Read the model definition and answer for the solid it produces. Units are mm, in the model's axes. A direction names the side the tool comes from. Round coordinates to 2 decimals unless told otherwise and drop trailing zeros. Write each loop counter-clockwise with the first axis right and the second up, starting at its lowest first coordinate (ties: lowest second). Pieces come first, ordered by that corner, then holes. Notation, with made-up numbers: (69.5, -13) - (117.5, -13) arc R8 ccw to (117.5, -6) - close; hole circle Ø6 at (59, -1.5). An arc over 180 degrees is marked (long way). Answer as CSV lines item,"result". Start each with the question number.
1) Find section C-C on x = 6. Determine the outline of the cut face in (y, z), then the cut area to 3 significant figures.
2) Each of these flat-tipped pins is pushed along its axis until it touches: pin 1 (2 mm diameter, centred on x = 5.5, y = -3, fed in from -Z); pin 2 (12 mm diameter, centred on y = 3.5, z = -15, fed in from +X). Where does it stop, or does it pass through?
3) Find section D-D on z = -14. Determine the outline of the cut face in (x, y), then the cut area to 3 significant figures.
4) Consider line 1 along X through (y, z) = (-2, 0.4); line 2 along Z through (x, y) = (7.25, -2.75); line 3 along Y through (x, z) = (3.25, -16.75). Determine where each line is inside the solid, lowest interval first.
5) Which of the six approach directions +Z, -Z, +X, -X, +Y, -Y give full straight-line access (tool end or side, diameter ignored) to faces 1 (the cylindrical face through (0.14, 9.43, 0.4)), 2 (the flat face through (0, 9, -10))?
6) For a pull along X with two mould halves and no side action, classify faces 3 (the cylindrical face through (1.952, -1.566, 0.493)), 4 (the flat face through (7.5, -7.5, 0.5)), 5 (the flat face through (0, 1, 0)), 6 (the flat face through (-7.5, -7.5, 0.5)) as +X half, -X half, draft (parallel to the pull), parting line (faces both ways), or undercut.
7) Find section B-B on y = -2. Determine the outline of the cut face in (x, z), then the cut area to 3 significant figures.
8) Find section A-A on x = 0. Determine the outline of the cut face in (y, z).
Autodesk Inventor part; units mm, degrees
ref_plane "YZ Plane" through (0, 0, 0) normal (1, 0, 0) x (0, 1, 0)
ref_plane "XZ Plane" through (0, 0, 0) normal (0, 1, 0) x (-1, 0, 0)
ref_plane "XY Plane" through (0, 0, 0) normal (0, 0, 1) x (1, 0, 0)
sketch "Sketch1" plane through (0, 0, 0) normal (0, 0, 1) x (1, 0, 0)
  line L0 (-10, -10) -> (10, -10)
  line L1 (10, -10) -> (10, 10)
  line L2 (10, 10) -> (-10, 10)
  line L3 (-10, 10) -> (-10, -10)
  line L4 (-10, -10) -> (10, 10) construction
  line L5 (10, -10) -> (-10, 10) construction
  point P0 (0, 0)
  dimension "d0" = 20
  dimension "d1" = 20
extrude "Plate1" add sketch "Sketch1" along normal blind 1
sketch "Sketch2" plane through (10, 9, 1) normal (0, 1, 0) x (-1, 0, 0)
  line L0 (20, 0) -> (0, 0)
  line L1 (0, 0) -> (0, -20)
  line L2 (0, -20) -> (20, -20)
  line L3 (20, -20) -> (20, 0)
edge flange "Flange1" height 20 angle 90 thickness 1 bend radius 1 thickness toward (0, 1, 0) relief tear relief width 1 relief depth 0.5 edges at (0, 10, 0) wall of the first edge with corners at (-10, 9, 1) (10, 9, 1) (10, 9, -19) (-10, 9, -19)
bend "Bend1"
corner "Corner1"
sketch "Sketch3" plane through (0, 0, 1) normal (0, 0, 1) x (1, 0, 0)
  line L0 (5, -10) -> (-5, -10)
  point P0 (0, -2)
  point P1 (0, -2)
  point P2 (10, -10)
  point P3 (-10, -10)
  point P4 (0, -10)
  dimension "d23" = 8
chamfer "Corner Chamfer1" distance 5 angle 45 2 edges at (10, -10, 0.5) (-10, -10, 0.5)
hole "Hole1" at (0, -2, 1) direction (0, 0, -1) diameter 4 depth 1 tip angle 118
equation "\"d21\" = Thickness"
equation "\"d3\" = BendReliefWidth"
equation "\"d4\" = BendReliefDepth"
equation "\"d5\" = MinimumRemnant"
equation "\"d6\" = BendRadius"
equation "\"d9\" = BendRadius"
equation "\"d10\" = CornerReliefSize"
equation "\"d11\" = GapSize"
equation "\"d12\" = JacobiRadiusSize"
equation "\"BendRadius\" = Thickness"
equation "\"BendReliefWidth\" = Thickness"
equation "\"BendReliefDepth\" = 0.5 * Thickness"
equation "\"CornerReliefSize\" = 4 * Thickness"
equation "\"MinimumRemnant\" = 2 * Thickness"
equation "\"TransitionRadius\" = BendRadius"
equation "\"JacobiRadiusSize\" = BendRadius"
equation "\"GapSize\" = Thickness"
equation "\"d2\" = BendRadius"
Check values:
1,outline,"(-9, 0) - (8, 0) arc R1 cw to (9, -1) - (9, -19) - (10, -19) - (10, -1) arc R2 ccw to (8, 1) - (-9, 1) - close"
1,area,"37.4 mm^2"
2,pin 1,"stops at z = 0"
2,pin 2,"stops at x = 10"
3,outline,"(-10, 9) - (10, 9) - (10, 10) - (-10, 10) - close"
3,area,"20.0 mm^2"
4,line 1,"x = -10 to -2, 2 to 10"
4,line 2,"z = 0 to 1"
4,line 3,"y = 9 to 10"
5,face 1,"+Z, +X, -X, +Y"
5,face 2,"-Z, +X, -X, -Y"
6,face 3,"undercut"
6,face 4,"+X half"
6,face 5,"draft"
6,face 6,"-X half"
7,outline,"(-10, 0) - (-2, 0) - (-2, 1) - (-10, 1) - close; (2, 0) - (10, 0) - (10, 1) - (2, 1) - close"
7,area,"16.0 mm^2"
8,outline,"(-10, 0) - (-4, 0) - (-4, 1) - (-10, 1) - close; (0, 0) - (8, 0) arc R1 cw to (9, -1) - (9, -19) - (10, -19) - (10, -1) arc R2 ccw to (8, 1) - (0, 1) - close"
